from build123d import *

# Parameters (mm, degrees)
ESBO_O1_W                = 640
ESBO_O1_H                = 360
ESBO_O1_W_2              = 170
ESBO_O1_H_2              = 58
ESBO_O1_W_3              = 58
ESBO_O1_H_3              = 170
RESSALTO_EXTRUS_O1_DEPTH = 20
ESBO_O2_R                = 4
CORTE_EXTRUS_O1_DEPTH    = 15


with BuildPart() as part:
    # Esboço1 → Ressalto-extrusão1 (new body)
    with BuildSketch(Plane.XY):
        with Locations((320, 180)):
            Rectangle(ESBO_O1_W, ESBO_O1_H)
        Polygon((215, 330), (425, 330), (425, 187.5), (215, 187.5), (215, 257), align=None, mode=Mode.SUBTRACT)
        with Locations((115, 301)):
            Rectangle(ESBO_O1_W_2, ESBO_O1_H_2, mode=Mode.SUBTRACT)
        with Locations((59, 115)):
            Rectangle(ESBO_O1_W_3, ESBO_O1_H_3, mode=Mode.SUBTRACT)
        with Locations((581, 245)):
            Rectangle(ESBO_O1_W_3, ESBO_O1_H_3, mode=Mode.SUBTRACT)
        Polygon((200, 257), (30, 257), (30, 215), (88, 215), (103, 215), (103, 30), (200, 30), align=None, mode=Mode.SUBTRACT)
        Polygon((425, 88), (425, 30), (215, 30), (215, 172.5), (425, 172.5), (425, 103), align=None, mode=Mode.SUBTRACT)
        with Locations((525, 59)):
            Rectangle(ESBO_O1_W_2, ESBO_O1_H_2, mode=Mode.SUBTRACT)
        Polygon((440, 103), (610, 103), (610, 145), (537, 145), (537, 160), (537, 330), (440, 330), align=None, mode=Mode.SUBTRACT)
    extrude(amount=RESSALTO_EXTRUS_O1_DEPTH)

    # Esboço2 → Corte-extrusão1 (cut)
    with BuildSketch(Plane(origin=(0, 0, 0), x_dir=(-1, 0, 0), z_dir=(0, 0, -1))):
        with Locations((-179, 337.5)):
            Circle(ESBO_O2_R)
        with Locations((-179, 264.5)):
            Circle(ESBO_O2_R)
        with Locations((-22.5, 179)):
            Circle(ESBO_O2_R)
        with Locations((-95.5, 179)):
            Circle(ESBO_O2_R)
        with Locations((-461, 95.5)):
            Circle(ESBO_O2_R)
        with Locations((-461, 22.5)):
            Circle(ESBO_O2_R)
        with Locations((-544.5, 181)):
            Circle(ESBO_O2_R)
        with Locations((-617.5, 181)):
            Circle(ESBO_O2_R)
    extrude(amount=-CORTE_EXTRUS_O1_DEPTH, mode=Mode.SUBTRACT)


solid = part.part
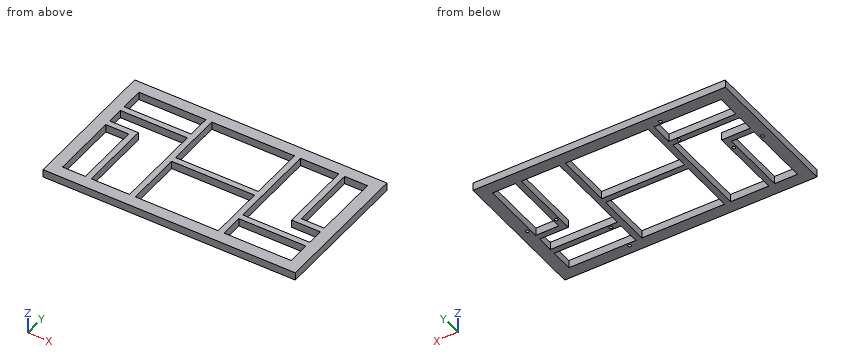
Geometry: final body of the model. Coordinates: model frame, mm. Give positions to 0.01 mm unless a question says otherwise; leave off trailing zeros. Order: outer loops, then holes, each group sorted by start corner. A loop starts at its lowest first (then second) coordinate and runs counter-clockwise, first axis right, second up. Notation, with made-up numbers: (30, 30) -> (65, 30) arc R28 ccw to (65, 61) -> close; hole circle Ø11 at (56, -9.5). An arc over 180 degrees is marked (long way). Write each question's results on one line, items separated by ' | '.
1) Line query: line 1 along X through (y, z) = (66.5, 4); line 2 along Y through (x, z) = (267, 8.5); line 3 along Y through (x, z) = (573, 9.5). Output: solid intervals per line, ascending.
Geometry says:
line 1: x = 0 to 30, 88 to 103, 200 to 215, 425 to 440, 610 to 640 | line 2: y = 0 to 30, 172.5 to 187.5, 330 to 360 | line 3: y = 0 to 30, 88 to 103, 145 to 160, 330 to 360
2) Cut plane B-B (x = 147.5). Output: boundary loops of the cut face in (y, z), and give its area (3 significant figures).
Geometry says:
outline: (0, 0) -> (30, 0) -> (30, 20) -> (0, 20) -> close; (257, 0) -> (272, 0) -> (272, 20) -> (257, 20) -> close; (330, 0) -> (360, 0) -> (360, 20) -> (330, 20) -> close | area: 1,500 mm²
3) Cut plane A-A (y = 81.5). Output: boundary loops of the cut face in (x, z), and give its area (3 significant figures).
Geometry says:
outline: (0, 0) -> (30, 0) -> (30, 20) -> (0, 20) -> close; (88, 0) -> (103, 0) -> (103, 20) -> (88, 20) -> close; (200, 0) -> (215, 0) -> (215, 20) -> (200, 20) -> close; (425, 0) -> (440, 0) -> (440, 20) -> (425, 20) -> close; (610, 0) -> (640, 0) -> (640, 20) -> (610, 20) -> close | area: 2,100 mm²
4) First-contact query: pin 1 Ø6.5 at (x, y) = (545, 181) entering from -Z. Flat tip, straight axial feed; report the tip coordinate or a pass-through.
Geometry says:
pin 1: stops at z = 15
5) Cut plane C-C (z = 6.5). Give the number of separate pieces and of enclosed holes in the cut face, and give its area (3 significant figures).
Geometry says:
separate pieces: 1 | enclosed holes: 16 | area: 80,500 mm²
